Read the model definition and answer for the solid it produces. Units are mm, in the model's axes. Face numbers are marked on the shaded views. Coordinates: 2 decimals unless noted, no trailing zeros. Write each loop counter-clockwise with the first axis right and the second up, starting at its lowest first coordinate (ties: lowest second). Pieces come first, ordered by that corner, then holes.
Item 1: Straight lines are drawn through the part: probe 1 along Y at (x, z) = (0, -4.5); probe 2 along Y at (x, z) = (0, -5.5); probe 3 along Z at (x, y) = (9.5, 9.5). For each, find the intervals that lie inside material, in ascending order.
Item 2: Section A-A (x = 0) is taken. Give the vertices of the cut face in (y, z).
Item 3: Section D-D (y = 9) is taken. Give the vertices of the cut face in (x, z), then the cut area to 3 significant figures.
Item 4: Determine the mould class of the marked faces 1, 2 and 3 for opening direction X: released by +X, released by -X, zero draft, split by the parting line, or undercut.
Item 5: Section C-C (z = -3) is taken. Give the vertices of the cut face in (x, y).
Item 6: Each of these flat-tipped pins is pushed along its axis until it touches: P1, Ø2, axis at x = -10.5, y = 6.5, coming from the +Z side; P2, Ø1.5, axis at x = -11, z = -1.5, coming from the +Y side; P3, Ø1.5, axis at x = 6, z = -5, coming from the -Y side. Where does it stop, or does it pass through?
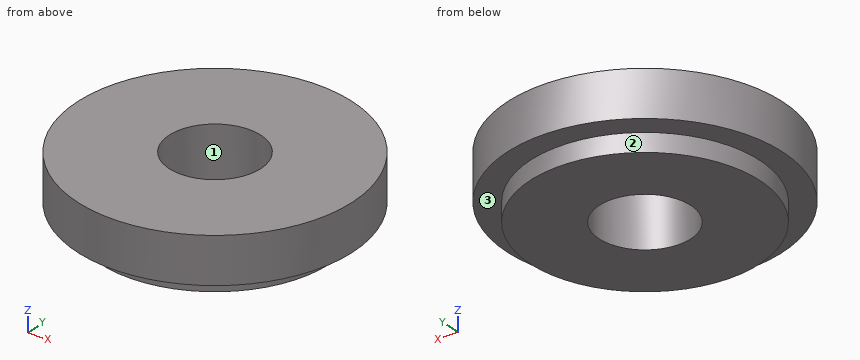
Autodesk Inventor part; units mm, degrees
ref_plane "YZ Plane" through (0, 0, 0) normal (1, 0, 0) x (0, 1, 0)
ref_plane "XZ Plane" through (0, 0, 0) normal (0, 1, 0) x (-1, 0, 0)
ref_plane "XY Plane" through (0, 0, 0) normal (0, 0, 1) x (1, 0, 0)
sketch "Sketch2" plane through (0, 0, 0) normal (0, 0, 1) x (1, 0, 0)
  circle A0 centre (0, 0) radius 15
  dimension "d0" = 30
extrude "Extrusion1" add sketch "Sketch2" against normal blind 5
sketch "Sketch3" plane through (0, 0, 0) normal (0, 0, 1) x (1, 0, 0)
  circle A0 centre (0, 0) radius 12.5
  dimension "d3" = 25
extrude "Extrusion2" add sketch "Sketch3" against normal blind 7
sketch "Sketch4" plane through (0, 0, 0) normal (0, 0, 1) x (1, 0, 0)
  circle A0 centre (0, 0) radius 5
  dimension "d6" = 10
extrude "Extrusion3" cut sketch "Sketch4" against normal blind 7
equation "\"BendRadius\" = Thickness"
equation "\"BendReliefWidth\" = Thickness"
equation "\"BendReliefDepth\" = 0.5 * Thickness"
equation "\"CornerReliefSize\" = 4 * Thickness"
equation "\"MinimumRemnant\" = 2 * Thickness"
equation "\"TransitionRadius\" = BendRadius"
equation "\"JacobiRadiusSize\" = BendRadius"
equation "\"GapSize\" = Thickness"
properties part number "Bushing_beam_stempel_short"
Established:
1. probe 1: y = -15 to -5, 5 to 15
1. probe 2: y = -12.5 to -5, 5 to 12.5
1. probe 3: z = -5 to 0
2. outline: (-15, -5) - (-12.5, -5) - (-12.5, -7) - (-5, -7) - (-5, 0) - (-15, 0) - close; (5, -7) - (12.5, -7) - (12.5, -5) - (15, -5) - (15, 0) - (5, 0) - close
3. outline: (-12, -5) - (-8.67, -5) - (-8.67, -7) - (8.67, -7) - (8.67, -5) - (12, -5) - (12, 0) - (-12, 0) - close
3. area: 155 mm2
4. face 1: undercut
4. face 2: split by the parting line
4. face 3: zero draft
5. outline: circle Ø30 at (0, 0); hole circle Ø10 at (0, 0)
6. P1: stops at z = 0
6. P2: stops at y = 10.95
6. P3: stops at y = -14.05
